The model under review builds one solid part; all positions refer to its coordinate system, in mm. Face numbers are marked on the shaded views. A direction names the side the tool comes from. Round coordinates to 2 decimals unless told otherwise and drop trailing zeros. Order: outer loops, then holes, each group sorted by start corner. A loop starts at its lowest first (then second) coordinate and runs counter-clockwise, first axis right, second up. Notation, with made-up numbers: (43, 34) - (59, 34) arc R32 cw to (59, 66) - close; hole circle Ø7 at (75.5, 62.5). An arc over 180 degrees is marked (long way). One line per question, with ' | ' between items. Start each with the question number.
Item 1: Add section B-B on x = -2.25. State the section outline as (y, z) points, and give its area (3 significant figures).
Item 2: Insertion check: pin 1 Ø0.7 at (x, z) = (0, 1.5) entering from -Y; pin 2 Ø0.5 at (x, z) = (1, 1) entering from +Y; pin 3 Ø0.5 at (y, z) = (-3.5, 1.5) entering from +X. Each pin has a flat end and moves straight along its axis. Give the tip position at first contact, or say it passes through.
Item 3: For L1, parallel to X at y = -3.5, z = 1.15; L2, parallel to Z at x = -1.5, y = 3.5; L3, parallel to Y at x = 0.75, z = 1.05, list the stretches that pass through material, from the lowest coordinate up. Write a range as [from, to].
Item 4: Tool access review of the marked faces 1 and 2: name each direction out of +Z, -Z, +X, -X, +Y, -Y from which nothing blocks a thin tool from reaching the whole face with its end or side.
Item 5: Add section A-A on y = -5.5. State the section outline as (x, z) points.
Item 6: Add section C-C on z = 0.25. State the section outline as (x, y) points.
Item 7: Add section D-D on z = 1.6. State the section outline as (x, y) points, and give its area (3 significant figures).
Item 8: Draft analysis for pull direction Y (two halves, no side actions). For the marked faces 3, 4, 5 and 6, state which applies: +Y half, -Y half, draft (parallel to the pull), parting line (faces both ways), or undercut.
from build123d import *

# Parameters (mm, degrees)
SKIZZE1_W                       = 6.6
SKIZZE1_H                       = 6.2
LINEAR_AUSTRAGEN1_DEPTH         = 2.4
FASE2_SIZE                      = 0.6
SKIZZE2_W                       = 0.9
SKIZZE2_H                       = 0.6
SKIZZE3_W                       = 0.9
SKIZZE3_H                       = 0.6
LINEAR_AUSTRAGEN2_DEPTH         = 1
SKIZZE4_W                       = 5.4
SKIZZE4_H                       = 0.6
LINEAR_AUSTRAGEN3_DEPTH         = 0.8
SKIZZE5_W                       = 3.4
SKIZZE5_H                       = 0.6
SCHNITT_LINEAR_AUSTRAGEN1_DEPTH = 0.3
FASE3_SIZE                      = 0.3
FASE4_SIZE                      = 0.1


with BuildPart() as part:
    # Skizze1 → Linear austragen1 (new body)
    with BuildSketch(Plane.XY):
        Rectangle(SKIZZE1_W, SKIZZE1_H)
    extrude(amount=LINEAR_AUSTRAGEN1_DEPTH)

    # Fase2
    fase2_edges = [part.edges().sort_by_distance(p)[0] for p in [
        (-3.3, 3.1, 1.2),
        (3.3, 3.1, 1.2),
    ]]
    chamfer(fase2_edges, length=FASE2_SIZE)

    # Austragung1: sweep along a curve in space
    with BuildLine() as austragung1_path:
        Line((2.3, -3.1, 1.4), (2.3, -4.3, 1.4))
        ThreePointArc((2.3, -4.3, 1.4), (2.3, -4.653553391, 1.253553391), (2.3, -4.8, 0.9))
        Line((2.3, -4.8, 0.9), (2.3, -4.8, 0.8))
        ThreePointArc((2.3, -4.8, 0.8), (2.3, -4.946446609, 0.446446609), (2.3, -5.3, 0.3))
        Line((2.3, -5.3, 0.3), (2.3, -6.2, 0.3))
    # Skizze2 → Austragung1 (sweep)
    with BuildSketch(Plane.XZ.offset(3.1)):
        with Locations((2.3, 1.4)):
            Rectangle(SKIZZE2_W, SKIZZE2_H)
    austragung1 = sweep(path=austragung1_path.line)

    # Spiegeln1: Austragung1 across plane
    add(austragung1.mirror(Plane(origin=(0, 0, 0), x_dir=(0, 0, 1), z_dir=(1, 0, 0))))

    # Skizze3 → Linear austragen2 (add)
    with BuildSketch(Plane.XZ.offset(3.1)):
        with Locations((0, 1.4)):
            Rectangle(SKIZZE3_W, SKIZZE3_H)
    extrude(amount=LINEAR_AUSTRAGEN2_DEPTH)

    # Skizze4 → Linear austragen3 (add)
    with BuildSketch(Plane(origin=(0, 3.1, 0), x_dir=(-1, 0, 0), z_dir=(0, 1, 0))):
        with Locations((0, 0.3)):
            Rectangle(SKIZZE4_W, SKIZZE4_H)
    extrude(amount=LINEAR_AUSTRAGEN3_DEPTH)

    # Skizze5 → Schnitt-Linear austragen1 (cut)
    with BuildSketch(Plane(origin=(0, 3.9, 0), x_dir=(-1, 0, 0), z_dir=(0, 1, 0))):
        with Locations((0, 0.3)):
            Rectangle(SKIZZE5_W, SKIZZE5_H)
    extrude(amount=-SCHNITT_LINEAR_AUSTRAGEN1_DEPTH, mode=Mode.SUBTRACT)

    # Fase3
    fase3_edges = [part.edges().sort_by_distance(p)[0] for p in [
        (-2.7, 3.9, 0.3),
        (2.7, 3.9, 0.3),
    ]]
    chamfer(fase3_edges, length=FASE3_SIZE)

    # Fase4
    fase4_edges = [part.edges().sort_by_distance(p)[0] for p in [
        (0, -3.1, 2.4),
        (-3.3, -0.3, 2.4),
        (-3, 2.8, 2.4),
        (0, 3.1, 2.4),
        (3, 2.8, 2.4),
        (3.3, -0.3, 2.4),
    ]]
    chamfer(fase4_edges, length=FASE4_SIZE)


solid = part.part
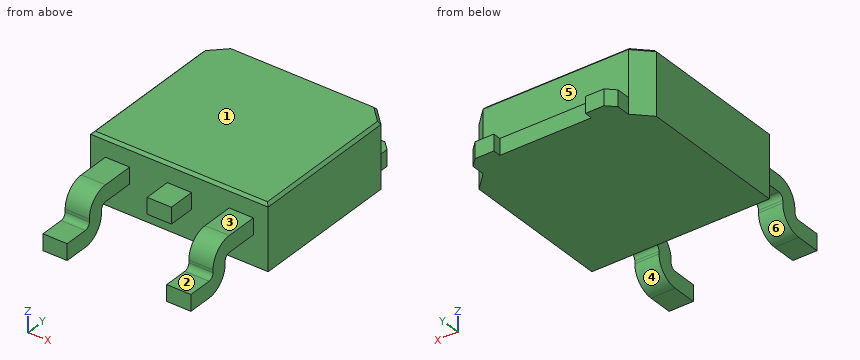
Determined:
1) outline: (-6.2, 0) - (-5.3, 0) arc R0.8 ccw to (-4.5, 0.8) - (-4.5, 0.9) arc R0.2 cw to (-4.3, 1.1) - (-3.1, 1.1) - (-3.1, 0) - (3.9, 0) - (3.9, 0.6) - (3.1, 0.6) - (3.1, 2.3) - (3, 2.4) - (-3, 2.4) - (-3.1, 2.3) - (-3.1, 1.7) - (-4.3, 1.7) arc R0.8 ccw to (-5.1, 0.9) - (-5.1, 0.8) arc R0.2 cw to (-5.3, 0.6) - (-6.2, 0.6) - close | area: 17.6 mm2
2) pin 1: y = -4.1 | pin 2: y = 3.1 | pin 3: x = 2.75
3) L1: [-2.75, -1.85], [-0.45, 0.45], [1.85, 2.75] | L2: [0, 0.6] | L3: [-3.1, 3.1]
4) face 1: +Z, +X, -X, +Y, -Y | face 2: +Z, +X, -X, -Y
5) outline: (-2.75, 0) - (-1.85, 0) - (-1.85, 0.6) - (-2.75, 0.6) - close; (1.85, 0) - (2.75, 0) - (2.75, 0.6) - (1.85, 0.6) - close
6) outline: (-3.3, -3.1) - (3.3, -3.1) - (3.3, 2.5) - (2.7, 3.1) - (2.7, 3.6) - (2.4, 3.9) - (1.7, 3.9) - (1.7, 3.6) - (-1.7, 3.6) - (-1.7, 3.9) - (-2.4, 3.9) - (-2.7, 3.6) - (-2.7, 3.1) - (-3.3, 2.5) - close; (-2.75, -6.2) - (-1.85, -6.2) - (-1.85, -4.72) - (-2.75, -4.72) - close; (1.85, -6.2) - (2.75, -6.2) - (2.75, -4.72) - (1.85, -4.72) - close
7) outline: (-3.3, -3.1) - (-2.75, -3.1) - (-2.75, -4.69) - (-1.85, -4.69) - (-1.85, -3.1) - (-0.45, -3.1) - (-0.45, -4.1) - (0.45, -4.1) - (0.45, -3.1) - (1.85, -3.1) - (1.85, -4.69) - (2.75, -4.69) - (2.75, -3.1) - (3.3, -3.1) - (3.3, 2.5) - (2.7, 3.1) - (-2.7, 3.1) - (-3.3, 2.5) - close | area: 44.3 mm2
8) face 3: draft | face 4: undercut | face 5: +Y half | face 6: undercut
